from build123d import *

# Parameters (mm, degrees)
SKETCH1_R           = 13.545312508
SKETCH1_R_2         = 12.7
SKETCH1_R_3         = 2.749999961
BOSS_EXTRUDE1_DEPTH = 6.35


with BuildPart() as part:
    # Sketch1 → Boss-Extrude1 (new body)
    with BuildSketch(Plane(origin=(0, 0, 0), x_dir=(1, 0, 0), z_dir=(0, 1, 0))):
        with BuildLine():
            Line((141.475775265, 8.956769201), (78.494677297, 118.043230799))
            ThreePointArc((78.494677297, 118.043230799), (71.937867169, 124.600040926), (62.981097968, 127))
            Line((62.981097968, 127), (-62.981097968, 127))
            ThreePointArc((-62.981097968, 127), (-71.937867169, 124.600040926), (-78.494677297, 118.043230799))
            Line((-78.494677297, 118.043230799), (-141.475775265, 8.956769201))
            ThreePointArc((-141.475775265, 8.956769201), (-143.875734339, 0), (-141.475775265, -8.956769201))
            Line((-141.475775265, -8.956769201), (-78.494677297, -118.043230799))
            ThreePointArc((-78.494677297, -118.043230799), (-71.937867169, -124.600040926), (-62.981097968, -127))
            Line((-62.981097968, -127), (62.981097968, -127))
            ThreePointArc((62.981097968, -127), (71.937867169, -124.600040926), (78.494677297, -118.043230799))
            Line((78.494677297, -118.043230799), (141.475775265, -8.956769201))
            ThreePointArc((141.475775265, -8.956769201), (143.875734339, 0), (141.475775265, 8.956769201))
        make_face()
        with Locations(Location((-58.65878735, 101.6, 0), (0, 0, 270))):
            Circle(SKETCH1_R, mode=Mode.SUBTRACT)
        with Locations(Location((-58.65878735, -101.6, 0), (0, 0, 270))):
            Circle(SKETCH1_R, mode=Mode.SUBTRACT)
        with Locations(Location((58.65878735, -101.6, 0), (0, 0, 270))):
            Circle(SKETCH1_R, mode=Mode.SUBTRACT)
        with Locations(Location((58.65878735, 101.6, 0), (0, 0, 270))):
            Circle(SKETCH1_R, mode=Mode.SUBTRACT)
        with Locations(Location((-117.317574699, 0, 0), (0, 0, 270))):
            Circle(SKETCH1_R_2, mode=Mode.SUBTRACT)
        with Locations(Location((117.317574699, 0, 0), (0, 0, 270))):
            Circle(SKETCH1_R_2, mode=Mode.SUBTRACT)
        with Locations(Location((-72.091982251, 78.333023923, 0), (0, 0, 270))):
            Circle(SKETCH1_R_3, mode=Mode.SUBTRACT)
        with Locations(Location((-31.792397547, 101.6, 0), (0, 0, 270))):
            Circle(SKETCH1_R_3, mode=Mode.SUBTRACT)
        with Locations(Location((31.792397547, 101.6, 0), (0, 0, 270))):
            Circle(SKETCH1_R_3, mode=Mode.SUBTRACT)
        with Locations(Location((72.091982251, 78.333023923, 0), (0, 0, 270))):
            Circle(SKETCH1_R_3, mode=Mode.SUBTRACT)
        with Locations(Location((-103.884379798, 23.266976077, 0), (0, 0, 270))):
            Circle(SKETCH1_R_3, mode=Mode.SUBTRACT)
        with Locations(Location((-103.884379798, -23.266976077, 0), (0, 0, 270))):
            Circle(SKETCH1_R_3, mode=Mode.SUBTRACT)
        with Locations(Location((-31.792397547, -101.6, 0), (0, 0, 270))):
            Circle(SKETCH1_R_3, mode=Mode.SUBTRACT)
        with Locations(Location((-72.091982251, -78.333023923, 0), (0, 0, 270))):
            Circle(SKETCH1_R_3, mode=Mode.SUBTRACT)
        with Locations(Location((103.884379798, -23.266976077, 0), (0, 0, 270))):
            Circle(SKETCH1_R_3, mode=Mode.SUBTRACT)
        with Locations(Location((103.884379798, 23.266976077, 0), (0, 0, 270))):
            Circle(SKETCH1_R_3, mode=Mode.SUBTRACT)
        with Locations(Location((72.091982251, -78.333023923, 0), (0, 0, 270))):
            Circle(SKETCH1_R_3, mode=Mode.SUBTRACT)
        with Locations(Location((31.792397547, -101.6, 0), (0, 0, 270))):
            Circle(SKETCH1_R_3, mode=Mode.SUBTRACT)
        with BuildLine():
            Line((82.816987915, 8.956769201), (49.165283622, 67.243230799))
            ThreePointArc((49.165283622, 67.243230799), (42.608473495, 73.800040926), (33.651704293, 76.2))
            Line((33.651704293, 76.2), (-33.651704293, 76.2))
            ThreePointArc((-33.651704293, 76.2), (-42.608473495, 73.800040926), (-49.165283622, 67.243230799))
            Line((-49.165283622, 67.243230799), (-82.816987915, 8.956769201))
            ThreePointArc((-82.816987915, 8.956769201), (-85.216946989, 0), (-82.816987915, -8.956769201))
            Line((-82.816987915, -8.956769201), (-49.165283622, -67.243230799))
            ThreePointArc((-49.165283622, -67.243230799), (-42.608473495, -73.800040926), (-33.651704293, -76.2))
            Line((-33.651704293, -76.2), (33.651704293, -76.2))
            ThreePointArc((33.651704293, -76.2), (42.608473495, -73.800040926), (49.165283622, -67.243230799))
            Line((49.165283622, -67.243230799), (82.816987915, -8.956769201))
            ThreePointArc((82.816987915, -8.956769201), (85.216946989, 0), (82.816987915, 8.956769201))
        make_face(mode=Mode.SUBTRACT)
        with BuildLine():
            Line((-24.555367407, 114.3), (24.555367407, 114.3))
            ThreePointArc((24.555367407, 114.3), (22.267397547, 101.6), (24.555367407, 88.9))
            Line((24.555367407, 88.9), (-24.555367407, 88.9))
            ThreePointArc((-24.555367407, 88.9), (-22.267397547, 101.6), (-24.555367407, 114.3))
        make_face(mode=Mode.SUBTRACT)
        with BuildLine():
            Line((-86.709019949, 78.415571974), (-111.264387356, 35.884428026))
            ThreePointArc((-111.264387356, 35.884428026), (-99.121879798, 31.515868048), (-89.2673421, 23.184428026))
            Line((-89.2673421, 23.184428026), (-64.711974693, 65.715571974))
            ThreePointArc((-64.711974693, 65.715571974), (-76.854482251, 70.084131952), (-86.709019949, 78.415571974))
        make_face(mode=Mode.SUBTRACT)
        with BuildLine():
            Line((-89.2673421, -23.184428026), (-64.711974693, -65.715571974))
            ThreePointArc((-64.711974693, -65.715571974), (-76.854482251, -70.084131952), (-86.709019949, -78.415571974))
            Line((-86.709019949, -78.415571974), (-111.264387356, -35.884428026))
            ThreePointArc((-111.264387356, -35.884428026), (-99.121879798, -31.515868048), (-89.2673421, -23.184428026))
        make_face(mode=Mode.SUBTRACT)
        with BuildLine():
            Line((-24.555367407, -88.9), (24.555367407, -88.9))
            ThreePointArc((24.555367407, -88.9), (22.267397547, -101.6), (24.555367407, -114.3))
            Line((24.555367407, -114.3), (-24.555367407, -114.3))
            ThreePointArc((-24.555367407, -114.3), (-22.267397547, -101.6), (-24.555367407, -88.9))
        make_face(mode=Mode.SUBTRACT)
        with BuildLine():
            Line((89.2673421, -23.184428026), (64.711974693, -65.715571974))
            ThreePointArc((64.711974693, -65.715571974), (76.854482251, -70.084131952), (86.709019949, -78.415571974))
            Line((86.709019949, -78.415571974), (111.264387356, -35.884428026))
            ThreePointArc((111.264387356, -35.884428026), (99.121879798, -31.515868048), (89.2673421, -23.184428026))
        make_face(mode=Mode.SUBTRACT)
        with BuildLine():
            Line((64.711974693, 65.715571974), (89.2673421, 23.184428026))
            ThreePointArc((89.2673421, 23.184428026), (99.121879798, 31.515868048), (111.264387356, 35.884428026))
            Line((111.264387356, 35.884428026), (86.709019949, 78.415571974))
            ThreePointArc((86.709019949, 78.415571974), (76.854482251, 70.084131952), (64.711974693, 65.715571974))
        make_face(mode=Mode.SUBTRACT)
    extrude(amount=BOSS_EXTRUDE1_DEPTH)


solid = part.part
Geometry check sheet. Reference: the model listing, model coordinates, mm. A direction names the side the tool comes from. Coordinates: 2 decimals unless noted, no trailing zeros. Write each loop counter-clockwise with the first axis right and the second up, starting at its lowest first coordinate (ties: lowest second). Pieces come first, ordered by that corner, then holes. Notation, with made-up numbers: (-22, 47.5) -> (17, 47.5) arc R27 ccw to (17, 76.5) -> close; hole circle Ø9 at (-8.5, 67.5). An arc over 180 degrees is marked (long way). One line per question, with ' | ' between items.
1. Draft check along X on faces 3 (the flat face through (-109.544, 3.131, -64.264)), 4 (the cylindrical face through (72.051, 3.131, -124.534)), 5 (the cylindrical face through (-22.268, 3.131, -101.418)), 6 (the flat face through (-2, 6.35, -86)). Enter one of: +X half, -X half, draft (parallel to the pull), parting line (faces both ways), or undercut.
Answers:
face 3: -X half | face 4: +X half | face 5: undercut | face 6: draft
2. Cross-section at D-D on y = 5.25. State how many separate pieces and enclosed holes the cut face has, and give its area (3 significant figures).
Answers:
separate pieces: 1 | enclosed holes: 25 | area: 25,100 mm²
3. Thickness scan on probe 1 along X at (y, z) = (2.75, -101.6); probe 2 along Z at (x, y) = (6, 0.5); probe 3 along X at (y, z) = (6, 44.5). Record the ranges inside material, lowest first. Write a range as from..to.
Answers:
probe 1: x = -87.99..-72.2, -45.11..-34.54, -29.04..-22.27, 22.27..29.04, 34.54..45.11, 72.2..87.99 | probe 2: z = -127..-114.3, -88.9..-76.2, 76.2..88.9, 114.3..127 | probe 3: x = -120.95..-106.29, -76.96..-62.3, 62.3..76.96, 106.29..120.95
4. Set-up check for faces 1 (the cylindrical face through (42.722, 3.131, -73.734)), 2 (the flat face through (-1, 3, 127)): record each of +Z, -Z, +X, -X, +Y, -Y from which the full face is reachable in a straight line by a thin tool's end or side.
Answers:
face 1: +Y, -Y | face 2: +Z, +X, -X, +Y, -Y
5. Depth check by flat-ended pin: pin 1 Ø24.5 at (x, z) = (-58.66, -101.6) entering from -Y; pin 2 Ø1 at (y, z) = (2, 27) entering from -X; pin 3 Ø6.5 at (x, z) = (-31.79, -101.6) entering from -Y; pin 4 Ø1.5 at (y, z) = (5, -78) entering from +X. Enter the tip coordinate at first touch or a pass-through.
Answers:
pin 1: passes through | pin 2: stops at x = -131.35 | pin 3: stops at y = 0 | pin 4: stops at x = 102.05
6. Cross-section at C-C on x = -120.5. Record the cut outline in (y, z).
Answers:
outline: (0, -45.29) -> (6.35, -45.29) -> (6.35, -12.29) -> (0, -12.29) -> close; (0, 12.29) -> (6.35, 12.29) -> (6.35, 45.29) -> (0, 45.29) -> close
7. Cross-section at A-A on z = 0. Record the cut outline in (x, y).
Answers:
outline: (-143.88, 0) -> (-130.02, 0) -> (-130.02, 6.35) -> (-143.88, 6.35) -> close; (-104.62, 0) -> (-85.22, 0) -> (-85.22, 6.35) -> (-104.62, 6.35) -> close; (85.22, 0) -> (104.62, 0) -> (104.62, 6.35) -> (85.22, 6.35) -> close; (130.02, 0) -> (143.88, 0) -> (143.88, 6.35) -> (130.02, 6.35) -> close
8. Cross-section at B-B on x = -2.5. Record the cut outline in (y, z), and give its area (3 significant figures).
Answers:
outline: (0, -127) -> (6.35, -127) -> (6.35, -114.3) -> (0, -114.3) -> close; (0, -88.9) -> (6.35, -88.9) -> (6.35, -76.2) -> (0, -76.2) -> close; (0, 76.2) -> (6.35, 76.2) -> (6.35, 88.9) -> (0, 88.9) -> close; (0, 114.3) -> (6.35, 114.3) -> (6.35, 127) -> (0, 127) -> close | area: 323 mm²
